from build123d import *

# Parameters (mm, degrees)
SKETCH1_W                                  = 95.4
SKETCH1_H                                  = 76
BOSS_EXTRUDE1_DEPTH                        = 13
SKETCH2_R                                  = 3.5
CUT_EXTRUDE1_DEPTH                         = 14
MIRROR1_AT_THE_SECOND_PLANE_COPY_1_SKETC_R = 3.5
MIRROR1_AT_THE_SECOND_PLANE_COPY_1_DEPTH   = 14
SKETCH3_W                                  = 105.4
SKETCH3_H                                  = 86
SKETCH3_W_2                                = 95.4
SKETCH3_H_2                                = 76
BOSS_EXTRUDE2_DEPTH                        = 20
SKETCH3_4_W                                = 105.4
SKETCH3_4_H                                = 20
BOSS_EXTRUDE3_DEPTH                        = 60
CBORE_FOR_M6_SHCS1_D                       = 7
CBORE_FOR_M6_SHCS1_CBORE_D                 = 11
CBORE_FOR_M6_SHCS1_CBORE_DEPTH             = 6
FILLET1_R                                  = 15


with BuildPart() as part:
    # Sketch1 → Boss-Extrude1 (new body)
    with BuildSketch(Plane(origin=(0, 0, 0), x_dir=(1, 0, 0), z_dir=(0, 1, 0))):
        Rectangle(SKETCH1_W, SKETCH1_H)
    extrude(amount=BOSS_EXTRUDE1_DEPTH)

    # Sketch2 → Cut-Extrude1 (cut, through all)
    with BuildSketch(Plane(origin=(0, 13, 0), x_dir=(1, 0, 0), z_dir=(0, 1, 0))):
        with Locations((-34.1, 31)):
            Circle(SKETCH2_R)
        with Locations((-9.7, 26.5)):
            Circle(SKETCH2_R)
    cut_extrude1 = extrude(amount=-CUT_EXTRUDE1_DEPTH, mode=Mode.SUBTRACT)

    # Mirror1: Cut-Extrude1 across plane
    add(cut_extrude1.mirror(Plane(origin=(0, 0, 0), x_dir=(0, 0, 1), z_dir=(1, 0, 0))), mode=Mode.SUBTRACT)

    # Mirror1 at the second plane: Cut-Extrude1 across plane
    add(cut_extrude1.mirror(Plane.XY), mode=Mode.SUBTRACT)

    # Mirror1 at the second plane copy 1 sketc → Mirror1 at the second plane copy 1 (cut, through all)
    with BuildSketch(Plane(origin=(0, 13, 0), x_dir=(-1, 0, 0), z_dir=(0, 1, 0))):
        with Locations((-34.1, 31)):
            Circle(MIRROR1_AT_THE_SECOND_PLANE_COPY_1_SKETC_R)
        with Locations((-9.7, 26.5)):
            Circle(MIRROR1_AT_THE_SECOND_PLANE_COPY_1_SKETC_R)
    extrude(amount=-MIRROR1_AT_THE_SECOND_PLANE_COPY_1_DEPTH, mode=Mode.SUBTRACT)

    # Sketch3 → Boss-Extrude2 (add)
    with BuildSketch(Plane(origin=(0, 13, 0), x_dir=(1, 0, 0), z_dir=(0, 1, 0))):
        Rectangle(SKETCH3_W, SKETCH3_H)
        Rectangle(SKETCH3_W_2, SKETCH3_H_2, mode=Mode.SUBTRACT)
    extrude(amount=-BOSS_EXTRUDE2_DEPTH)

    # Sketch3<4> → Boss-Extrude3 (add)
    with BuildSketch(Plane(origin=(0, 13, 0), x_dir=(1, 0, 0), z_dir=(0, 1, 0))):
        with Locations((0, 53)):
            Rectangle(SKETCH3_4_W, SKETCH3_4_H)
    extrude(amount=-BOSS_EXTRUDE3_DEPTH)

    # CBORE for M6 SHCS1 (through all)
    with Locations(Plane(origin=(37.5, -37, -43), x_dir=(1, 0, 0), z_dir=(0, 0, 1))):
        with Locations((0, 0), (-75, 0)):
            CounterBoreHole(CBORE_FOR_M6_SHCS1_D / 2, CBORE_FOR_M6_SHCS1_CBORE_D / 2, CBORE_FOR_M6_SHCS1_CBORE_DEPTH)

    # Fillet1
    fillet1_edges = [part.edges().sort_by_distance(p)[0] for p in [
        (-52.7, -47, -53),
        (52.7, -47, -53),
    ]]
    fillet(fillet1_edges, radius=FILLET1_R)


solid = part.part
The listing builds one solid part. Answer for the finished solid, in the listing's coordinates (mm). A direction names the side the tool comes from. Coordinates: 2 decimals unless noted, no trailing zeros. Loops run counter-clockwise (first coordinate to the right, second up) from the corner with the lowest first, then second, coordinate; pieces in that order, holes last.
1) Flat-ended cylindrical pins translate along their axes: pin 1 Ø5.5 at (x, z) = (9.7, -26.5) entering from +Y; pin 2 Ø10 at (x, z) = (-25, -5.5) entering from -Y; pin 3 Ø5.5 at (x, y) = (-39.5, -39) entering from +Z. Find the tip coordinate at first contact, or state that the pin passes through.
2) Determine the mould class of faces 4 (the face through (52.7, 1, -21)), 5 (the face through (-1, -47, -53)), 6 (the face through (-1, 0, -1)) for opening direction X: pulls with the +X half, pulls with the -X half, needs draft (parallel to the pull), parting line crosses it, or undercut.
3) A tool of negligible diameter and unlimited length cuts with its end or side. For faces 1 (the face through (-1, -3, -38)), 2 (the face through (-43, -37, -46)), 3 (the face through (0, -7, 41)), from which of +Z, -Z, +X, -X, +Y, -Y can it reach the whole face along a straight path? Write none if from no direction.
4) Find section D-D on z = 0.5. Write down the section's boundary in (x, y).
5) Find section C-C on x = 9.7. Write down the section's boundary in (y, z), then the cut area to 3 significant figures.
6) Find section B-B on y = 1.5. Give the number of separate pieces and of enclosed holes in the cut face, then the cut area to 3 significant figures.
7) Find section A-A on z = -45.5. Write down the section's boundary in (x, y).
8) Find the intervals of material crossed by L1, parallel to Z at x = -25, y = -1.5; L2, parallel to Z at x = 9.7, y = 9.5; L3, parallel to Y at x = 37, z = -47, in increasing order.
Values:
1. pin 1: passes through
1. pin 2: stops at y = 0
1. pin 3: stops at z = -43
2. face 4: pulls with the +X half
2. face 5: needs draft
2. face 6: undercut
3. face 1: -Y
3. face 2: +Z
3. face 3: +Z, +X, -X, -Y
4. outline: (-52.7, -7) - (-47.7, -7) - (-47.7, 0) - (47.7, 0) - (47.7, -7) - (52.7, -7) - (52.7, 13) - (-52.7, 13) - close
5. outline: (-47, -63) - (13, -63) - (13, -30) - (0, -30) - (0, -38) - (-7, -38) - (-7, -43) - (-47, -43) - close; (-7, 38) - (0, 38) - (0, 30) - (13, 30) - (13, 43) - (-7, 43) - close; (0, -23) - (13, -23) - (13, 23) - (0, 23) - close
5. area: 2,210 mm2
6. separate pieces: 1
6. enclosed holes: 8
6. area: 10,900 mm2
7. outline: (-52.7, -32) arc R15 ccw to (-37.7, -47) - (37.7, -47) arc R15 ccw to (52.7, -32) - (52.7, 13) - (-52.7, 13) - close; hole circle Ø11 at (-37.5, -37); hole circle Ø11 at (37.5, -37)
8. L1: z = -63 to -38, 38 to 43
8. L2: z = -63 to -30, -23 to 23, 30 to 43
8. L3: y = -47 to -42.48, -31.52 to 13
